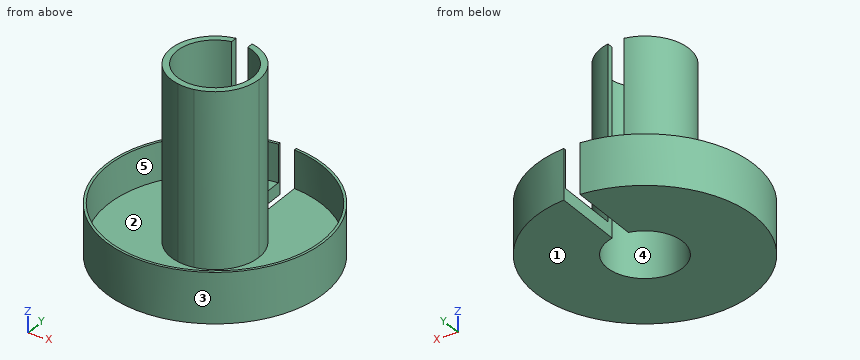
from build123d import *

# Parameters (mm, degrees)
F1_DEPTH = 25.4
F2_DEPTH = 6.35
F3_DEPTH = 93.98


with BuildPart() as f1:
    # F0 (on Top) → F1 (new body)
    with BuildSketch(Plane.XY):
        with BuildLine():
            ThreePointArc((-1.1352293447, 35.2420264333), (34.3776264235, 18.1213738464), (48.7757706553, -18.579758459))
            ThreePointArc((48.7757706553, -18.579758459), (-41.9003616501, -58.1566142273), (-9.2632293447, 35.2420264333))
            Line((-9.2632293447, 35.2420264333), (-9.2632293447, 36.515558302))
            ThreePointArc((-9.2632293447, 36.515558302), (-42.7990587659, -59.0552183391), (50.0457706553, -18.579758459))
            ThreePointArc((50.0457706553, -18.579758459), (35.2762305353, 19.0200709621), (-1.1352293447, 36.515558302))
            Line((-1.1352293447, 36.515558302), (-1.1352293447, 35.2420264333))
        make_face()
    extrude(amount=F1_DEPTH)

    # F0 (on Top) → F2 (join)
    with BuildSketch(Plane.XY):
        with BuildLine():
            ThreePointArc((-9.2632293447, 35.2420264333), (-41.9003616501, -58.1566142273), (48.7757706553, -18.579758459))
            ThreePointArc((48.7757706553, -18.579758459), (34.3776264235, 18.1213738464), (-1.1352293447, 35.2420264333))
            Line((-1.1352293447, 35.2420264333), (-1.1352293447, 3.2705168024))
            ThreePointArc((-1.1352293447, 3.2705168024), (11.8927720741, -4.3736290601), (17.0257706553, -18.579758459))
            ThreePointArc((17.0257706553, -18.579758459), (11.8927720741, -32.785887858), (-1.1352293447, -40.4300337205))
            Line((-1.1352293447, -40.4300337205), (-1.1352293447, -67.4839898818))
            Line((-1.1352293447, -67.4839898818), (-9.2632293447, -67.4839898818))
            Line((-9.2632293447, -67.4839898818), (-9.2632293447, -40.4300337205))
            ThreePointArc((-9.2632293447, -40.4300337205), (-27.4242293447, -18.579758459), (-9.2632293447, 3.2705168024))
            Line((-9.2632293447, 3.2705168024), (-9.2632293447, 35.2420264333))
        make_face()
        with BuildLine():
            ThreePointArc((17.0257706553, -18.579758459), (11.8927720741, -4.3736290601), (-1.1352293447, 3.2705168024))
            Line((-1.1352293447, 3.2705168024), (-1.1352293447, 0.0317004843))
            ThreePointArc((-1.1352293447, 0.0317004843), (9.6385888911, -6.6323047554), (13.8507706553, -18.579758459))
            ThreePointArc((13.8507706553, -18.579758459), (9.6385888911, -30.5272121626), (-1.1352293447, -37.1912174024))
            Line((-1.1352293447, -37.1912174024), (-1.1352293447, -40.4300337205))
            ThreePointArc((-1.1352293447, -40.4300337205), (11.8927720741, -32.785887858), (17.0257706553, -18.579758459))
        make_face()
        with BuildLine():
            Line((-9.2632293447, -37.1912174024), (-9.2632293447, -40.4300337205))
            ThreePointArc((-9.2632293447, -40.4300337205), (-5.1992293447, -40.804758459), (-1.1352293447, -40.4300337205))
            Line((-1.1352293447, -40.4300337205), (-1.1352293447, -37.1912174024))
            ThreePointArc((-1.1352293447, -37.1912174024), (-5.1992293447, -37.629758459), (-9.2632293447, -37.1912174024))
        make_face()
        with BuildLine():
            Line((-9.2632293447, 0.0317004843), (-9.2632293447, 3.2705168024))
            ThreePointArc((-9.2632293447, 3.2705168024), (-27.4242293447, -18.579758459), (-9.2632293447, -40.4300337205))
            Line((-9.2632293447, -40.4300337205), (-9.2632293447, -37.1912174024))
            ThreePointArc((-9.2632293447, -37.1912174024), (-24.2492293447, -18.579758459), (-9.2632293447, 0.0317004843))
        make_face()
        with BuildLine():
            ThreePointArc((-1.1352293447, -40.4300337205), (-5.1992293447, -40.804758459), (-9.2632293447, -40.4300337205))
            Line((-9.2632293447, -40.4300337205), (-9.2632293447, -67.4839898818))
            Line((-9.2632293447, -67.4839898818), (-1.1352293447, -67.4839898818))
            Line((-1.1352293447, -67.4839898818), (-1.1352293447, -40.4300337205))
        make_face()
    extrude(amount=F2_DEPTH)

    # F0 (on Top) → F3 (join)
    with BuildSketch(Plane.XY):
        with BuildLine():
            ThreePointArc((17.0257706553, -18.579758459), (11.8927720741, -4.3736290601), (-1.1352293447, 3.2705168024))
            Line((-1.1352293447, 3.2705168024), (-1.1352293447, 0.0317004843))
            ThreePointArc((-1.1352293447, 0.0317004843), (9.6385888911, -6.6323047554), (13.8507706553, -18.579758459))
            ThreePointArc((13.8507706553, -18.579758459), (9.6385888911, -30.5272121626), (-1.1352293447, -37.1912174024))
            Line((-1.1352293447, -37.1912174024), (-1.1352293447, -40.4300337205))
            ThreePointArc((-1.1352293447, -40.4300337205), (11.8927720741, -32.785887858), (17.0257706553, -18.579758459))
        make_face()
        with BuildLine():
            Line((-9.2632293447, -37.1912174024), (-9.2632293447, -40.4300337205))
            ThreePointArc((-9.2632293447, -40.4300337205), (-5.1992293447, -40.804758459), (-1.1352293447, -40.4300337205))
            Line((-1.1352293447, -40.4300337205), (-1.1352293447, -37.1912174024))
            ThreePointArc((-1.1352293447, -37.1912174024), (-5.1992293447, -37.629758459), (-9.2632293447, -37.1912174024))
        make_face()
        with BuildLine():
            Line((-9.2632293447, 0.0317004843), (-9.2632293447, 3.2705168024))
            ThreePointArc((-9.2632293447, 3.2705168024), (-27.4242293447, -18.579758459), (-9.2632293447, -40.4300337205))
            Line((-9.2632293447, -40.4300337205), (-9.2632293447, -37.1912174024))
            ThreePointArc((-9.2632293447, -37.1912174024), (-24.2492293447, -18.579758459), (-9.2632293447, 0.0317004843))
        make_face()
    extrude(amount=F3_DEPTH)


solid = f1.part
Here's how the part is built. I have some questions about the finished solid (model axes, mm). Face numbers are marked on the shaded views. A direction names the side the tool comes from. Round coordinates to 2 decimals unless told otherwise and drop trailing zeros. Write each loop counter-clockwise with the first axis right and the second up, starting at its lowest first coordinate (ties: lowest second). Pieces come first, ordered by that corner, then holes. Notation, with made-up numbers: (14, -9) -> (63, -9) arc R12 ccw to (63, 1) -> close; hole circle Ø6 at (37.25, 67.25). An arc over 180 degrees is marked (long way). One line per item, written item: value.
1) Suppose I cut it at B-B on y = -10.5. List the corners of the cut face in (x, z) for me.
Filled sheet:
outline: (-59.85, 0) -> (-22.45, 0) -> (-22.45, 93.98) -> (-25.9, 93.98) -> (-25.9, 6.35) -> (-58.57, 6.35) -> (-58.57, 25.4) -> (-59.85, 25.4) -> close; (12.05, 0) -> (49.45, 0) -> (49.45, 25.4) -> (48.17, 25.4) -> (48.17, 6.35) -> (15.51, 6.35) -> (15.51, 93.98) -> (12.05, 93.98) -> close
2) If I drill on line 1 (X direction, y = -29, z = 17); line 2 (Z direction, x = -42, y = -16); line 3 (Y direction, x = 37, z = 7), over which ranges is the centre line in solid material (lowest first)? Write a range as [from, to].
Filled sheet:
line 1: x = [-59.45, -58.16], [-24.83, -21.15], [10.75, 14.43], [47.76, 49.05]
line 2: z = [0, 6.35]
line 3: y = [-54.23, -52.23], [15.07, 17.07]
3) Suppose I cut it at C-C on x = 11. List the corners of the cut face in (y, z) for me, plus the area to 3 significant figures.
Filled sheet:
outline: (-71.4, 0) -> (-28.6, 0) -> (-28.6, 93.98) -> (-33.8, 93.98) -> (-33.8, 6.35) -> (-70.07, 6.35) -> (-70.07, 25.4) -> (-71.4, 25.4) -> close; (-8.56, 0) -> (34.24, 0) -> (34.24, 25.4) -> (32.91, 25.4) -> (32.91, 6.35) -> (-3.36, 6.35) -> (-3.36, 93.98) -> (-8.56, 93.98) -> close
area: 1,500 mm2
4) Suppose I cut it at A-A on z = 21. List the corners of the cut face in (x, y) for me (3 decimals).
Filled sheet:
outline: (-9.263, 0.032) -> (-9.263, 3.271) arc R22.225 ccw (long way) to (-1.135, 3.271) -> (-1.135, 0.032) arc R19.05 cw (long way) to start; (-9.263, 35.242) -> (-9.263, 36.516) arc R55.245 ccw (long way) to (-1.135, 36.516) -> (-1.135, 35.242) arc R53.975 cw (long way) to start
5) We'd pull the mould along Y, two halves only. Please class the marked faces 1, 2 and 3: released by +Y, released by -Y, zero draft, split by the parting line, or undercut.
Filled sheet:
face 1: zero draft
face 2: undercut
face 3: split by the parting line
6) For the marked faces 4 and 5, which set-ups out of +Z, -Z, +X, -X, +Y, -Y let a thin tool reach every point of the face, with its end or its side?
Filled sheet:
face 4: +Z, -Z
face 5: +Z
7) Suppose I cut it at D-D on z = 73. List the corners of the cut face in (x, y) for me (3 decimals), plus the area to 3 significant figures.
Filled sheet:
outline: (-9.263, 0.032) -> (-9.263, 3.271) arc R22.225 ccw (long way) to (-1.135, 3.271) -> (-1.135, 0.032) arc R19.05 cw (long way) to start
area: 386 mm2
8) I'm going to push flat-ended pins straight in: pin 1 Ø5 at (x, z) = (-38, 24.5) entering from +Y; pin 2 Ø4 at (y, z) = (5, 25.5) entering from +X; pin 3 Ø8 at (x, y) = (-42.5, -24) entering from +Z. Where does each tip first touch, or does it pass through?
Filled sheet:
pin 1: stops at y = 27.61
pin 2: stops at x = 45.66
pin 3: stops at z = 6.35
